from build123d import *

# Parameters (mm, degrees)
MAIN_DEPTH                   = 35
SIDECUT_DEPTH                = 51
SIDECUT_DEPTH_BACK           = 1
SKETCH5_W                    = 40
SKETCH5_H                    = 50.207972894
CENTRALCUT_DEPTH             = 38.370465934
SKETCH3_R                    = 1.6
MAKERBEAMFIXHOLES_DEPTH      = 1
MAKERBEAMFIXHOLES_DEPTH_BACK = 47
ROLLERSUPPORTHOLES_DEPTH     = 22.5
LPATTERN1_COUNT              = 5
LPATTERN1_PITCH              = 10


with BuildPart() as part:
    # Sketch1 → Main (new body, symmetric)
    with BuildSketch(Plane.XY):
        Polygon((50, 45), (50, 40), (42.245330322, 40), (6.689774766, 0), (0, 0), (40, 45), (43.55, 45), (43.55, 46), (46.45, 46), (46.45, 45), align=None)
    extrude(amount=MAIN_DEPTH, both=True)

    # Sketch2 → SideCut (cut, two sides)
    with BuildSketch(Plane(origin=(0, 12.071067812, 0), x_dir=(0, 0, 1), z_dir=(1, 0, 0))) as sidecut_sk:
        Polygon((-35, -32.928932188), (-25, 12.071067812), (-35, 12.071067812), align=None)
        Polygon((35, -32.928932188), (35, 12.071067812), (25, 12.071067812), align=None)
    extrude(amount=SIDECUT_DEPTH, mode=Mode.SUBTRACT)
    extrude(sidecut_sk.sketch, amount=-SIDECUT_DEPTH_BACK, mode=Mode.SUBTRACT)

    # Sketch5 → CentralCut (cut, through all)
    with BuildSketch(Plane(origin=(0, 0, 0), x_dir=(0, 0, 1), z_dir=(-0.747409319, 0.664363839, 0))):
        with Locations((0, 30.103986447)):
            Rectangle(SKETCH5_W, SKETCH5_H)
    extrude(amount=-CENTRALCUT_DEPTH, mode=Mode.SUBTRACT)

    # Sketch3 → MakerBeamFixHoles (cut, two sides)
    with BuildSketch(Plane(origin=(0, 46, 0), x_dir=(1, 0, 0), z_dir=(0, 1, 0))) as makerbeamfixholes_sk:
        with Locations((45, 25)):
            Circle(SKETCH3_R)
        with Locations((45, -25)):
            Circle(SKETCH3_R)
    extrude(amount=MAKERBEAMFIXHOLES_DEPTH, mode=Mode.SUBTRACT)
    extrude(makerbeamfixholes_sk.sketch, amount=-MAKERBEAMFIXHOLES_DEPTH_BACK, mode=Mode.SUBTRACT)

    # Sketch4 → RollerSupportHoles (cut, symmetric)
    with BuildSketch(Plane.XY):
        with BuildLine():
            Line((34.685089289, 39.020725451), (32.691997773, 36.778497494))
            Line((32.691997773, 36.778497494), (33.813111751, 35.781951736))
            ThreePointArc((33.813111751, 35.781951736), (35.930771487, 35.906519956), (35.806203267, 38.024179692))
            Line((35.806203267, 38.024179692), (34.685089289, 39.020725451))
        make_face()
    rollersupportholes = extrude(amount=ROLLERSUPPORTHOLES_DEPTH, both=True, mode=Mode.SUBTRACT)

    # LPattern1: RollerSupportHoles ×5
    with Locations(*[Vector(-0.664363839, -0.747409319, 0) * (i * LPATTERN1_PITCH) for i in range(1, LPATTERN1_COUNT)]):
        add(rollersupportholes, mode=Mode.SUBTRACT)


solid = part.part
Here's how the part is built. I have some questions about the finished solid (model axes, mm). A direction names the side the tool comes from. Give positions to 0.01 mm unless a question says otherwise; leave off trailing zeros. Order: outer loops, then holes, each group sorted by start corner. A loop starts at its lowest first (then second) coordinate and runs counter-clockwise, first axis right, second up. Notation, with made-up numbers: (28.25, 73) -> (59.25, 73) arc R13 cw to (59.25, 77) -> close; hole circle Ø1 at (21.25, -16). An arc over 180 degrees is marked (long way). One line per item, written item: value. Start each with the question number.
1. Imagine slicing it at D-D, the plane z = -28.5. List the corners of the cut face in (x, y) for me, plus the area to 3 significant figures.
2. Imagine slicing it at C-C, the plane x = 31. List the corners of the cut face in (y, z) for me (3 decimals).
3. We'd pull the mould along Z, two halves only. Please class faces 1 (the face through (24.883, 24.062, 30.347)), 2 (the face through (35.909, 35.882, -21.232)), 3 (the face through (24, 27, -23)): released by +Z, released by -Z, zero draft, split by the parting line, or undercut.
4. Will these pins go through, and if not, where does the flat tip stop? pin 1 Ø1.1 at (x, y) = (34.5, 36.5) entering from +Z; pin 2 Ø1.1 at (x, y) = (27.5, 29.5) entering from +Z; pin 3 Ø4 at (x, y) = (7.5, 7) entering from +Z.
5. Imagine slicing it at A-A, the plane x = 45. List the corners of the cut face in (y, z) for me.
6. For faces 4 (the face through (9.334, 5.986, -21.232)), 5 (the face through (5.164, 2.099, -0.28)), 6 (the face through (43.4, 43.04, 24.93)), which set-ups out of +Z, -Z, +X, -X, +Y, -Y let a thin tool reach every point of the face, with its end or its side?
7. Imagine slicing it at B-B, the plane y = 27. List the corners of the cut face in (x, z) for me, plus the area to 3 significant figures.
8. I need wall thicknesses on probe 1 along Z at (x, y) = (45, 44.35); probe 2 along Z at (x, y) = (45, 43); probe 3 along X at (y, z) = (42.6, -25). Which ranges of each line are inside material? Lowest first, please. Write a range as from..to.
Values follow:
1. outline: (14, 15.75) -> (20.69, 15.75) -> (42.25, 40) -> (50, 40) -> (50, 45) -> (46.45, 45) -> (46.45, 46) -> (43.55, 46) -> (43.55, 45) -> (40, 45) -> close
1. area: 226 mm2
2. outline: (27.349, -31.078) -> (34.875, -32.75) -> (34.875, -20) -> (27.349, -20) -> close; (27.349, 20) -> (34.875, 20) -> (34.875, 32.75) -> (27.349, 31.078) -> close
3. face 1: released by +Z
3. face 2: undercut
3. face 3: zero draft
4. pin 1: stops at z = 33.23
4. pin 2: stops at z = 31.68
4. pin 3: stops at z = 26.99
5. outline: (40, -33.89) -> (45, -35) -> (46, -35) -> (46, -26.6) -> (40, -26.6) -> close; (40, -23.4) -> (46, -23.4) -> (46, 23.4) -> (40, 23.4) -> close; (40, 26.6) -> (46, 26.6) -> (46, 35) -> (45, 35) -> (40, 33.89) -> close
6. face 4: none
6. face 5: +X, +Y
6. face 6: +Y, -Y
7. outline: (24, -31) -> (30.69, -31) -> (30.69, -20) -> (24, -20) -> close; (24, 20) -> (30.69, 20) -> (30.69, 31) -> (24, 31) -> close
7. area: 147 mm2
8. probe 1: z = -34.86..-26.6, -23.4..23.4, 26.6..34.86
8. probe 2: z = -34.56..-26.6, -23.4..23.4, 26.6..34.56
8. probe 3: x = 37.87..43.4, 46.6..50
